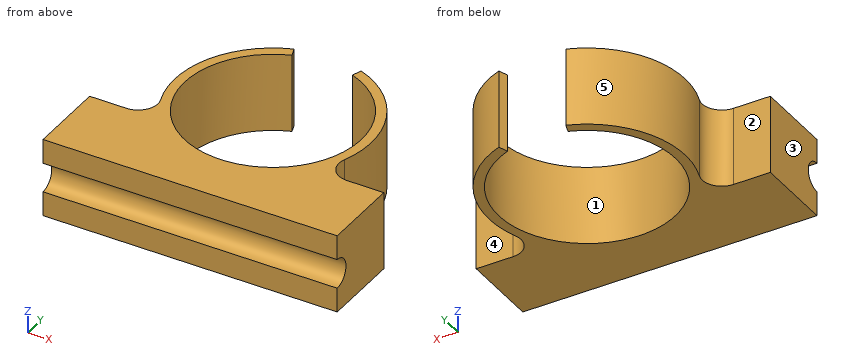
```python
from build123d import *

# Parameters (mm, degrees)
BOSS_EXTRUDE1_DEPTH = 8
SKETCH2_R           = 9
CUT_EXTRUDE1_DEPTH  = 35
SKETCH3_W           = 0.5
SKETCH3_H           = 1.875425002
CUT_EXTRUDE2_DEPTH  = 25
SKETCH4_R           = 1.5
CUT_EXTRUDE3_DEPTH  = 110
SKETCH6_W           = 5
SKETCH6_H           = 7.147198513
CUT_EXTRUDE4_DEPTH  = 10
FILLET1_R           = 0.5
SKETCH8_W           = 8
SKETCH8_H           = 3
BOSS_EXTRUDE2_DEPTH = 30
SKETCH9_R           = 9
CUT_EXTRUDE5_DEPTH  = 30
FILLET2_R           = 2
CUT_EXTRUDE7_DEPTH  = 30


with BuildPart() as part:
    # Sketch1 → Boss-Extrude1 (new body)
    with BuildSketch(Plane.XY):
        with BuildLine():
            Line((3.89007335, 2.5), (15, 2.5))
            Line((15, 2.5), (15, -2.5))
            Line((15, -2.5), (-15, -2.5))
            Line((-15, -2.5), (-15, 2.5))
            Line((-15, 2.5), (-3.89007335, 2.5))
            ThreePointArc((-3.89007335, 2.5), (0, 21.71234657), (3.89007335, 2.5))
        make_face()
    extrude(amount=BOSS_EXTRUDE1_DEPTH)

    # Sketch2 → Cut-Extrude1 (cut)
    with BuildSketch(Plane.XY.offset(8)):
        with Locations((0, 11.71234657)):
            Circle(SKETCH2_R)
    extrude(amount=-CUT_EXTRUDE1_DEPTH, mode=Mode.SUBTRACT)

    # Sketch3 → Cut-Extrude2 (cut)
    with BuildSketch(Plane(origin=(0, 0, 0), x_dir=(-1, 0, 0), z_dir=(0, 0, -1))):
        with Locations((0, 21.521483579)):
            Rectangle(SKETCH3_W, SKETCH3_H)
    extrude(amount=-CUT_EXTRUDE2_DEPTH, mode=Mode.SUBTRACT)

    # Sketch4 → Cut-Extrude3 (cut)
    with BuildSketch(Plane(origin=(15, 0, 0), x_dir=(0, 0, -1), z_dir=(1, 0, 0))):
        with Locations((-4, -2.5)):
            Circle(SKETCH4_R)
    extrude(amount=-CUT_EXTRUDE3_DEPTH, mode=Mode.SUBTRACT)

    # Sketch6 → Cut-Extrude4 (cut)
    with BuildSketch(Plane.XY.offset(8)):
        with Locations((0, 22.731746569)):
            Rectangle(SKETCH6_W, SKETCH6_H)
    extrude(amount=-CUT_EXTRUDE4_DEPTH, mode=Mode.SUBTRACT)

    # Fillet1
    fillet1_edges = [part.edges().sort_by_distance(p)[0] for p in [
        (-3.89007335, 2.5, 4),
        (3.89007335, 2.5, 4),
    ]]
    fillet(fillet1_edges, radius=FILLET1_R)

    # Sketch8 → Boss-Extrude2 (add)
    with BuildSketch(Plane.ZY.offset(15)):
        with Locations((4, 4)):
            Rectangle(SKETCH8_W, SKETCH8_H)
    extrude(amount=-BOSS_EXTRUDE2_DEPTH)

    # Sketch9 → Cut-Extrude5 (cut)
    with BuildSketch(Plane(origin=(0, 0, 0), x_dir=(-1, 0, 0), z_dir=(0, 0, -1))):
        with Locations((0, 11.71234657)):
            Circle(SKETCH9_R)
    extrude(amount=-CUT_EXTRUDE5_DEPTH, mode=Mode.SUBTRACT)

    # Fillet2
    fillet2_edges = [part.edges().sort_by_distance(p)[0] for p in [
        (-7.836245918, 5.5, 4),
        (7.836245918, 5.5, 4),
    ]]
    fillet(fillet2_edges, radius=FILLET2_R)

    # Sketch10 → Cut-Extrude7 (cut)
    with BuildSketch(Plane(origin=(0, 0, 0), x_dir=(-1, 0, 0), z_dir=(0, 0, -1))):
        with BuildLine():
            Line((0, 11.71234657), (3.420201433, 21.109272778))
            ThreePointArc((3.420201433, 21.109272778), (0, 24.529474212), (-3.420201433, 21.109272778))
            Line((-3.420201433, 21.109272778), (0, 11.71234657))
        make_face()
    extrude(amount=-CUT_EXTRUDE7_DEPTH, mode=Mode.SUBTRACT)


solid = part.part
```
The listing builds one solid part. Answer for the finished solid, in the listing's coordinates (mm). Face numbers are marked on the shaded views. A direction names the side the tool comes from. Give positions to 0.01 mm unless a question says otherwise; leave off trailing zeros. Write each loop counter-clockwise with the first axis right and the second up, starting at its lowest first coordinate (ties: lowest second). Pieces come first, ordered by that corner, then holes. Notation, with made-up numbers: (65, -4.5) -> (118, -4.5) arc R19 ccw to (118, 19.5) -> close; hole circle Ø9 at (34, 89). An arc over 180 degrees is marked (long way). Write item = value, one per line. Start each with the question number.
1) The part is cut by section C-C, the plane z = 3.25. Determine the outline of the cut face in (x, y).
2) The part is cut by section D-D, the plane y = 9.25. Determine the outline of the cut face in (x, z).
3) The part is cut by section A-A, the plane y = 18. Determine the outline of the cut face in (x, z), and give its area (3 significant figures).
4) Determine the mould class of the marked faces 3, 4 and 5 for opening direction Y: +Y half, -Y half, draft (parallel to the pull), parting line (faces both ways), or undercut.
5) Straight lines are drawn through the part: line 1 along X through (y, z) = (12, 0.5); line 2 along Y through (x, z) = (0, 2); line 3 along X through (y, z) = (17.5, 3.5). For each, find the intervals that lie inside material, in ascending order.
6) Which of the six approach directions +Z, -Z, +X, -X, +Y, -Y give full straight-line access (tool end or side, diameter ignored) to the marked faces 1 and 2?
7) The part is cut by section B-B, the plane x = -4.5. Determine the outline of the cut face in (y, z).
8) Each of these flat-tipped pins is pushed along its axis until it touches: pin 1 (3 mm diameter, centred on y = 15.5, z = 6.5, fed in from +X); pin 2 (3 mm diameter, centred on x = 13.5, z = 3.5, fed in from +Y); pin 3 (1 mm diameter, centred on x = -10, y = 5.5, fed in from -Z); pin 4 (4 mm diameter, centred on x = 4, y = 15, fed in from +Z). Where does it stop, or does it pass through?
Solutions:
q1.outline = (-15, -1.2) -> (15, -1.2) -> (15, 5.5) -> (11.24, 5.5) arc R2 cw to (9.36, 8.2) arc R10 ccw to (3.42, 21.11) -> (3.08, 20.17) arc R9 cw (long way) to (-3.08, 20.17) -> (-3.42, 21.11) arc R10 ccw to (-9.36, 8.2) arc R2 cw to (-11.24, 5.5) -> (-15, 5.5) -> close
q2.outline = (-9.69, 0) -> (-8.66, 0) -> (-8.66, 8) -> (-9.69, 8) -> close; (8.66, 0) -> (9.69, 0) -> (9.69, 8) -> (8.66, 8) -> close
q3.outline = (-7.78, 0) -> (-6.44, 0) -> (-6.44, 8) -> (-7.78, 8) -> close; (6.44, 0) -> (7.78, 0) -> (7.78, 8) -> (6.44, 8) -> close
q3.area = 21.4 mm²
q4.face_3 = draft
q4.face_4 = +Y half
q4.face_5 = undercut
q5.line_1 = -10 to -9, 9 to 10
q5.line_2 = -2.5 to 2.71
q5.line_3 = -8.15 to -6.89, 6.89 to 8.15
q6.face_1 = +Z, -Z
q6.face_2 = +Z, -Z, -X, +Y
q7.outline = (-2.5, 0) -> (3.92, 0) -> (3.92, 8) -> (-2.5, 8) -> (-2.5, 5.5) arc R1.5 cw to (-2.5, 2.5) -> close; (19.51, 0) -> (20.64, 0) -> (20.64, 8) -> (19.51, 8) -> close
q8.pin_1 = 9.73
q8.pin_2 = 5.5
q8.pin_3 = 0
q8.pin_4 = through
